Build history of the part. All positions in model axes, mm. A direction names the side the tool comes from. Round coordinates to 2 decimals unless told otherwise and drop trailing zeros. Write each loop counter-clockwise with the first axis right and the second up, starting at its lowest first coordinate (ties: lowest second). Pieces come first, ordered by that corner, then holes. Notation, with made-up numbers: M 69.5,60 L 74.5,60 A15 ccw 74.5,69 Z; hole C 85,-25.5 d1. An arc over 180 degrees is marked long. Write item = value, one per line. Start each with the question number.
Q1. Drop flat-ended pins along their axis: P1, Ø2.5, axis at y = 165, z = 210, coming from the +X side; P2, Ø3, axis at y = 165, z = 115, coming from the -X side. Give the stop position or say it passes through.
Q2. Tool access for faces 4 (the flat face through (-200, 165, 113)), 5 (the cylindrical face through (-65, 165, 25)): list every direction of +Z, -Z, +X, -X, +Y, -Y with a clear straight run to the whole face (end or side of a thin tool).
Q3. Band-saw the part on A-A on x = -37. Write the cut outline in (y, z), plus the area to 3 significant figures.
Q4. Probe L1, parallel to X at y = 165, z = 236; L2, parallel to Z at x = -198, y = 165; L3, parallel to X at y = 165.75, z = 182.5. List the from-to ranges inside material, lowest first.
Q5. Band-saw the part on C-C on z = 29. Write the cut outline in (x, y).
Q6. Band-saw the part on B-B on y = 168.5. State how many separate pieces and enclosed holes the cut face has, plus the area to 3 significant figures.
Q7. Pull direction Z, two halves, no side cores. Call faces 1 (the flat face through (-3, 160, 117)), 2 (the flat face through (-3, 165, 240)), 3 (the cylindrical face through (65, 165, 25)): released by +Z, released by -Z, zero draft, split by the parting line, or undercut.
```python
from build123d import *

# Parameters (mm, degrees)
SKETCH021_R               = 1.7
PAD019_DEPTH              = 20
SKETCH020_R               = 1.7
PAD018_DEPTH              = 20
SKETCH019_R               = 1.7
PAD017_DEPTH              = 20
CYLINDER038_R             = 1.7
CYLINDER038_DEPTH         = 61
CYLINDER038_PITCH_ANGLE   = 90
CYLINDER037_R             = 1.7
CYLINDER037_DEPTH         = 61
CYLINDER037_PITCH_ANGLE   = 90
CYLINDER036_R             = 1.7
CYLINDER036_DEPTH         = 61
CYLINDER036_PITCH_ANGLE   = 90
BOX001_W                  = 50
BOX001_H                  = 215
BOX001_DEPTH              = 115
CYLINDER039_R             = 1.7
CYLINDER039_DEPTH         = 61
CYLINDER039_PITCH_ANGLE   = 90
FUSION011_PLACEMENT_ANGLE = 90
SKETCH003_W               = 400
SKETCH003_H               = 250
SKETCH003_R               = 1.7
PAD003_DEPTH              = 10


with BuildPart() as pad019:
    # Sketch021 → Pad019 (new body)
    with BuildSketch(Plane(origin=(0, -75, 230), x_dir=(1, 0, 0), z_dir=(0, 0, 1))):
        with Locations((-150, 240)):
            Circle(SKETCH021_R)
        with Locations((150, 240)):
            Circle(SKETCH021_R)
        with Locations((0, 240)):
            Circle(SKETCH021_R)
    extrude(amount=PAD019_DEPTH)


with BuildPart() as pad018:
    # Sketch020 → Pad018 (new body)
    with BuildSketch(Plane.YZ.offset(-210)):
        with Locations((165, 210)):
            Circle(SKETCH020_R)
        with Locations((165, 115)):
            Circle(SKETCH020_R)
        with Locations((165, 20)):
            Circle(SKETCH020_R)
    extrude(amount=PAD018_DEPTH)


with BuildPart() as fusion013:
    # Sketch019 → Pad017 (new body)
    with BuildSketch(Plane.YZ.offset(210)):
        with Locations((165, 210)):
            Circle(SKETCH019_R)
        with Locations((165, 115)):
            Circle(SKETCH019_R)
        with Locations((165, 20)):
            Circle(SKETCH019_R)
    extrude(amount=-PAD017_DEPTH)

    # Fusion012: union Pad018
    add(pad018.part)

    # Fusion013: union Pad019
    add(pad019.part)


with BuildPart() as cylinder038:
    # Cylinder038 → Cylinder038 (new body)
    with BuildSketch(Plane.XY):
        Circle(CYLINDER038_R)
    extrude(amount=CYLINDER038_DEPTH)


with BuildPart() as cylinder038_1:
    # Cylinder038 pitch: moved
    add(cylinder038.part.rotate(Axis((0, 0, 0), (0, 1, 0)), CYLINDER038_PITCH_ANGLE))


with BuildPart() as cylinder038_2:
    # Cylinder038 placement: moved
    add(cylinder038_1.part.moved(Location((150, 112.5, 147.5))))


with BuildPart() as cylinder037:
    # Cylinder037 → Cylinder037 (new body)
    with BuildSketch(Plane.XY):
        Circle(CYLINDER037_R)
    extrude(amount=CYLINDER037_DEPTH)


with BuildPart() as cylinder037_1:
    # Cylinder037 pitch: moved
    add(cylinder037.part.rotate(Axis((0, 0, 0), (0, 1, 0)), CYLINDER037_PITCH_ANGLE))


with BuildPart() as cylinder037_2:
    # Cylinder037 placement: moved
    add(cylinder037_1.part.moved(Location((150, -37.5, 197.5))))


with BuildPart() as cylinder036:
    # Cylinder036 → Cylinder036 (new body)
    with BuildSketch(Plane.XY):
        Circle(CYLINDER036_R)
    extrude(amount=CYLINDER036_DEPTH)


with BuildPart() as cylinder036_1:
    # Cylinder036 pitch: moved
    add(cylinder036.part.rotate(Axis((0, 0, 0), (0, 1, 0)), CYLINDER036_PITCH_ANGLE))


with BuildPart() as cylinder036_2:
    # Cylinder036 placement: moved
    add(cylinder036_1.part.moved(Location((150, -37.5, 147.5))))


with BuildPart() as box001:
    # Box001 → Box001 (new body)
    with BuildSketch(Plane(origin=(150, -70, 115), x_dir=(1, 0, 0), z_dir=(0, 0, 1))):
        with Locations((25, 107.5)):
            Rectangle(BOX001_W, BOX001_H)
    extrude(amount=BOX001_DEPTH)


with BuildPart() as fusion011:
    # Cylinder039 → Cylinder039 (new body)
    with BuildSketch(Plane.XY):
        Circle(CYLINDER039_R)
    extrude(amount=CYLINDER039_DEPTH)


with BuildPart() as fusion011_1:
    # Cylinder039 pitch: moved
    add(fusion011.part.rotate(Axis((0, 0, 0), (0, 1, 0)), CYLINDER039_PITCH_ANGLE))


with BuildPart() as fusion011_2:
    # Cylinder039 placement: moved
    add(fusion011_1.part.moved(Location((150, 112.5, 197.5))))

    # Fusion011: union Cylinder038, Cylinder037, Cylinder036, Box001
    add(cylinder038_2.part)
    add(cylinder037_2.part)
    add(cylinder036_2.part)
    add(box001.part)


with BuildPart() as fusion011_3:
    # Fusion011 placement: moved
    add(fusion011_2.part.moved(Location((4.5, -41, -15))).rotate(Axis((4.5, -41, -15), (0, 0, 1)), FUSION011_PLACEMENT_ANGLE))


with BuildPart() as cut015:
    # Sketch003 → Pad003 (new body)
    with BuildSketch(Plane.XZ.offset(-170)):
        with Locations((0, 115)):
            Rectangle(SKETCH003_W, SKETCH003_H)
        with Locations((0, -5)):
            Circle(SKETCH003_R, mode=Mode.SUBTRACT)
        with Locations((-150, -5)):
            Circle(SKETCH003_R, mode=Mode.SUBTRACT)
        with Locations((150, -5)):
            Circle(SKETCH003_R, mode=Mode.SUBTRACT)
        with BuildLine():
            ThreePointArc((-50, 40), (-65, 25), (-50, 10))
            Line((-50, 10), (50, 10))
            ThreePointArc((50, 10), (65, 25), (50, 40))
            Line((-50, 40), (50, 40))
        make_face(mode=Mode.SUBTRACT)
    extrude(amount=PAD003_DEPTH)

    # Cut014: cut Fusion011
    add(fusion011_3.part, mode=Mode.SUBTRACT)

    # Cut015: cut Fusion013
    add(fusion013.part, mode=Mode.SUBTRACT)


solid = cut015.part
```
Conclusion:
q1.P1 = 190
q1.P2 = -190
q2.face_4 = +Z, -Z, -X, +Y, -Y
q2.face_5 = +Y, -Y
q3.outline = M 160,-10 L 170,-10 L 170,10 L 160,10 Z; M 160,40 L 170,40 L 170,240 L 160,240 Z
q3.area = 2,200 mm^2
q4.L1 = -200 to -151.7, -148.3 to -1.7, 1.7 to 148.3, 151.7 to 200
q4.L2 = -10 to 18.3, 21.7 to 113.3, 116.7 to 208.3, 211.7 to 240
q4.L3 = -200 to -109.7, -106.3 to 40.3, 43.7 to 200
q5.outline = M -200,160 L -64.46,160 L -64.46,170 L -200,170 Z; M 64.46,160 L 200,160 L 200,170 L 64.46,170 Z
q6.separate_pieces = 1
q6.enclosed_holes = 8
q6.area = 96,200 mm^2
q7.face_1 = zero draft
q7.face_2 = released by +Z
q7.face_3 = undercut
